Check sheet for the drawn part. Datum: minimum x, y, z corner. Units: mm. A direction names the side the tool comes from. Give positions to 0.01 mm unless a question says otherwise; leave off trailing zeros. Order: outer loops, then holes, each group sorted by start corner. A loop starts at its lowest first (then second) coordinate and runs counter-clockwise, first axis right, second up.
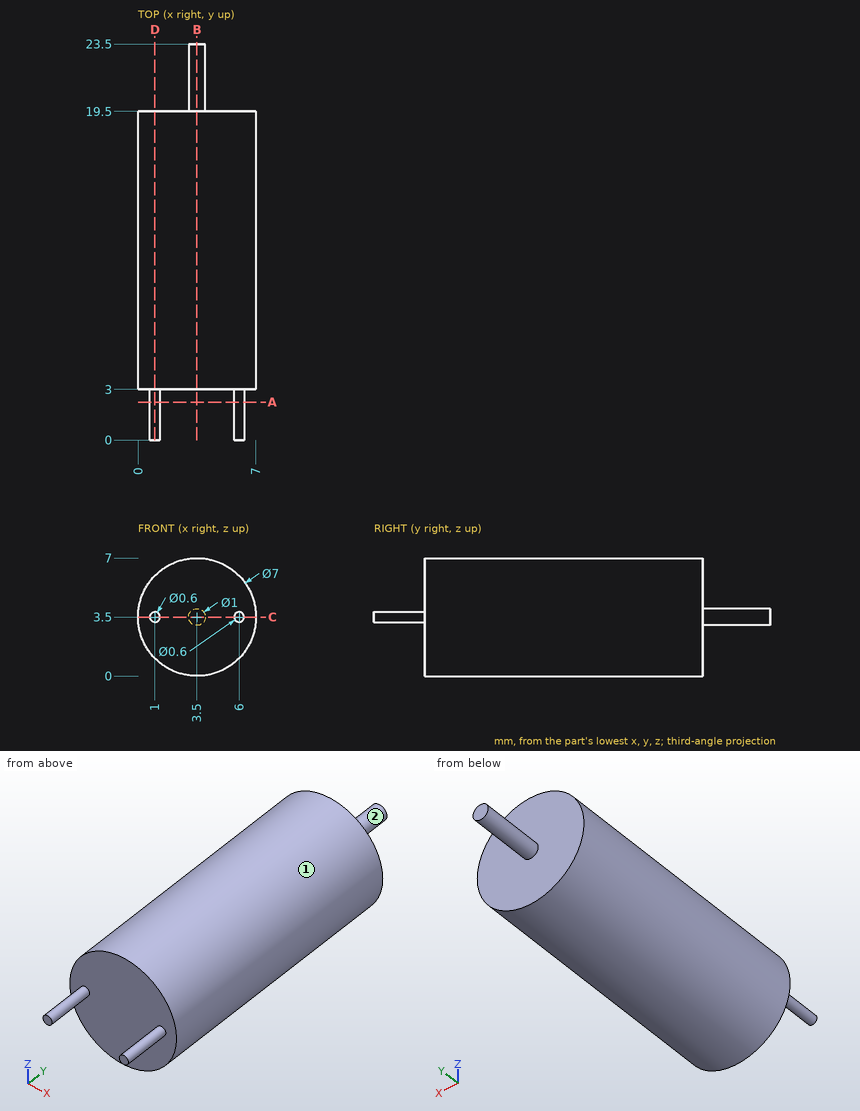
(1) Section check C-C, the plane z = 3.5. Enter the section's corners in (x, y), then the cut area to 3 significant figures.
Solved:
outline: (0, 3) - (0.7, 3) - (0.7, 0) - (1.3, 0) - (1.3, 3) - (5.7, 3) - (5.7, 0) - (6.3, 0) - (6.3, 3) - (7, 3) - (7, 19.5) - (4, 19.5) - (4, 23.5) - (3, 23.5) - (3, 19.5) - (0, 19.5) - close
area: 123 mm2
(2) Section check A-A, the plane y = 2.25. Enter the section's corners in (x, z), then the cut area to 3 significant figures.
Solved:
outline: circle Ø0.6 at (1, 3.5); circle Ø0.6 at (6, 3.5)
area: 0.565 mm2
(3) Section check B-B, the plane x = 3.5. Enter the section's corners in (y, z), then the cut area to 4 significant figures.
Solved:
outline: (3, 0) - (19.5, 0) - (19.5, 3) - (23.5, 3) - (23.5, 4) - (19.5, 4) - (19.5, 7) - (3, 7) - close
area: 119.5 mm2
(4) Section check D-D, the plane x = 1. Enter the section's corners in (y, z), then the cut area to 3 significant figures.
Solved:
outline: (0, 3.2) - (3, 3.2) - (3, 1.05) - (19.5, 1.05) - (19.5, 5.95) - (3, 5.95) - (3, 3.8) - (0, 3.8) - close
area: 82.6 mm2
(5) Scan lines: line 1 (Y direction, x = 2, z = 0.5); line 2 (Y direction, x = 3.25, z = 3.25); line 3 (X direction, y = 7.25, z = 6.25). Record each from-to range of solid material in increasing order.
Solved:
line 1: y = 3 to 19.5
line 2: y = 3 to 23.5
line 3: x = 1.33 to 5.67
(6) Go/stop test with flat-tipped pins: pin 1 (1 mm diameter, centred on y = 11.5, z = 1.5, fed in from +X); pin 2 (1.5 mm diameter, centred on x = 4.5, z = 6, fed in from -Y); pin 3 (1.5 mm diameter, centred on y = 6, z = 4.5, fed in from +X); pin 4 (3.5 mm diameter, centred on x = 5, z = 2, fed in from -Y). Record where each tip stops, or that it passes through.
Solved:
pin 1: stops at x = 6.66
pin 2: stops at y = 3
pin 3: stops at x = 6.99
pin 4: stops at y = 0
(7) Set-up check for the marked faces 1 and 2: record each of +Z, -Z, +X, -X, +Y, -Y from which the full face is reachable in a straight line by a thin tool's end or side.
Solved:
face 1: +Y, -Y
face 2: +Y
